```python
from build123d import *

# Parameters (mm, degrees)
F0_R     = 7.5
F0_R_2   = 3.556
F1_DEPTH = 9.525
F2_W     = 15
F2_H     = 6.604


with BuildPart() as f1:
    # F0 (on Top) → F1 (new body)
    with BuildSketch(Plane.XY):
        Circle(F0_R)
        Circle(F0_R_2, mode=Mode.SUBTRACT)
    extrude(amount=F1_DEPTH)

    # F2 (on Front) → F4 (revolve, cut)
    with BuildSketch(Plane.XZ):
        with Locations((11.564, 4.318)):
            Rectangle(F2_W, F2_H)
    revolve(axis=Axis((0, 0, 5.091826), (0, 0, 1)), mode=Mode.SUBTRACT)


solid = f1.part
```
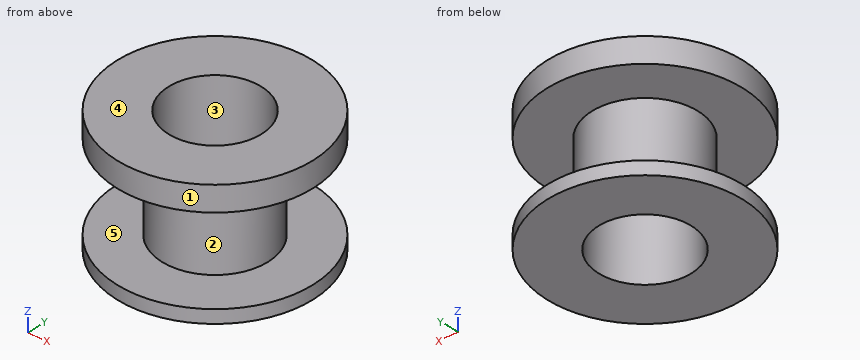
The listing builds one solid part. Answer for the finished solid, in the listing's coordinates (mm). Face numbers are marked on the shaded views. A direction names the side the tool comes from. Round coordinates to 2 decimals unless told otherwise and drop trailing zeros. Order: outer loops, then holes, each group sorted by start corner. A loop starts at its lowest first (then second) coordinate and runs counter-clockwise, first axis right, second up. Notation, with made-up numbers: (22.25, 0.25) - (80.25, 0.25) arc R18 ccw to (80.25, 30.25) - close; hole circle Ø2 at (72, 19.5). An arc over 180 degrees is marked (long way). Put each result on its own line as item: value. Start each with the question number.
(1) Find section C-C (z = 4). Give the vertices of the cut face in (x, y), plus the area to 3 significant figures.
(2) Find section B-B (x = 4.5). Give the vertices of the cut face in (y, z) (3 decimals).
(3) Find section A-A (y = 0). Give the vertices of the cut face in (x, z) (3 decimals), plus the area to 3 significant figures.
(4) Given P1, Ø1.5, axis at y = -2, z = 5, coming from the -X side; P2, Ø4, axis at x = 0, y = -1, coming from the +Z side; P3, Ø2, axis at y = -0.5, z = 2.5, coming from the +X side, each flat-ended and moving along its own axis, determine where each tip first touches the part or whether it passes through.
(5) Straight lines are drawn through the part: probe 1 along Z at (x, y) = (-3.5, 3.25) (3 decimals); probe 2 along Y at (x, z) = (0, 2.5); probe 3 along X at (y, z) = (0.5, 5.25). For each, find the intervals that lie inside material, in ascending order. Write a range as from..to.
(6) For the marked faces 1 and 2, determine the directions among +Z, -Z, +X, -X, +Y, -Y from which every point of the face is accessible in a straight line to the end or side of a thin tool.
(7) Determine the mould class of the marked faces 3, 4 and 5 for opening direction Z: released by +Z, released by -Z, zero draft, split by the parting line, or undercut.
Reply:
1. outline: circle Ø8.13 at (0, 0); hole circle Ø7.11 at (0, 0)
1. area: 12.2 mm^2
2. outline: (-6, 0) - (6, 0) - (6, 1.016) - (-6, 1.016) - close; (-6, 7.62) - (6, 7.62) - (6, 9.525) - (-6, 9.525) - close
3. outline: (-7.5, 0) - (-3.556, 0) - (-3.556, 9.525) - (-7.5, 9.525) - (-7.5, 7.62) - (-4.064, 7.62) - (-4.064, 1.016) - (-7.5, 1.016) - close; (3.556, 0) - (7.5, 0) - (7.5, 1.016) - (4.064, 1.016) - (4.064, 7.62) - (7.5, 7.62) - (7.5, 9.525) - (3.556, 9.525) - close
3. area: 29.8 mm^2
4. P1: x = -3.87
4. P2: through
4. P3: x = 4.06
5. probe 1: 0..1.016, 7.62..9.525
5. probe 2: -4.06..-3.56, 3.56..4.06
5. probe 3: -4.03..-3.52, 3.52..4.03
6. face 1: +Z, -Z
6. face 2: none
7. face 3: zero draft
7. face 4: released by +Z
7. face 5: undercut
